Check sheet for the modelled part. Datum: model origin and axes. Units: mm. A direction names the side the tool comes from. Round coordinates to 2 decimals unless told otherwise and drop trailing zeros. Write each loop counter-clockwise with the first axis right and the second up, starting at its lowest first coordinate (ties: lowest second). Pieces come first, ordered by that corner, then holes. Notation, with made-up numbers: (-34, -23.75) -> (9, -23.75) arc R25 ccw to (9, 3.25) -> close; hole circle Ø10 at (36, 20.5). An arc over 180 degrees is marked (long way). One line per item, written item: value.
from build123d import *

# Parameters (mm, degrees)
SKETCH1_R           = 27.5
SKETCH1_R_2         = 17.5
BOSS_EXTRUDE1_DEPTH = 5
SKETCH2_W           = 120
SKETCH2_H           = 6
BOSS_EXTRUDE2_DEPTH = 10
SKETCH3_W           = 5
SKETCH3_H           = 3
CUT_EXTRUDE1_DEPTH  = 140
CHAMFER1_SIZE       = 5


with BuildPart() as part:
    # Sketch1 → Boss-Extrude1 (new body)
    with BuildSketch(Plane.XY):
        Circle(SKETCH1_R)
        Circle(SKETCH1_R_2, mode=Mode.SUBTRACT)
    extrude(amount=BOSS_EXTRUDE1_DEPTH)

    # Sketch2 → Boss-Extrude2 (add)
    with BuildSketch(Plane.XY.offset(5)):
        with Locations((77.5, 0)):
            Rectangle(SKETCH2_W, SKETCH2_H)
    extrude(amount=-BOSS_EXTRUDE2_DEPTH)

    # Sketch3 → Cut-Extrude1 (cut)
    with BuildSketch(Plane.ZY.offset(-17.5)):
        with Locations((-2.5, 1.5)):
            Rectangle(SKETCH3_W, SKETCH3_H)
    extrude(amount=-CUT_EXTRUDE1_DEPTH, mode=Mode.SUBTRACT)

    # Chamfer1
    chamfer1_edges = [part.edges().sort_by_distance(p)[0] for p in [
        (17.5, -1.5, -5),
    ]]
    chamfer(chamfer1_edges, length=CHAMFER1_SIZE - 0.0001)  # a hair under: the kernel refuses the full size


solid = part.part
Item 1: Sectioned sample at B-B on y = -12. Enter the section's corners in (x, z).
Answer:
outline: (-24.74, 0) -> (-12.74, 0) -> (-12.74, 5) -> (-24.74, 5) -> close; (12.74, 0) -> (24.74, 0) -> (24.74, 5) -> (12.74, 5) -> close
Item 2: Mould release check, pull along X, two halves, no side actions. Record for faces 4 (the flat face through (137.5, -1, 1)), 5 (the cylindrical face through (-13.887, -10.648, 2.465)), 6 (the cylindrical face through (-27.475, 1.167, 2.465)), 7 (the flat face through (79, -1, -5)): pulls with the +X half, pulls with the -X half, needs draft (parallel to the pull), parting line crosses it, or undercut.
Answer:
face 4: pulls with the +X half
face 5: undercut
face 6: parting line crosses it
face 7: needs draft
Item 3: Sectioned sample at A-A on x = 0. Enter the section's corners in (y, z), and give its area (3 significant figures).
Answer:
outline: (-27.5, 0) -> (-17.5, 0) -> (-17.5, 5) -> (-27.5, 5) -> close; (17.5, 0) -> (27.5, 0) -> (27.5, 5) -> (17.5, 5) -> close
area: 100 mm^2
Item 4: Sectioned sample at D-D on x = 122.5. Enter the section's corners in (y, z).
Answer:
outline: (-3, -5) -> (0, -5) -> (0, 0) -> (3, 0) -> (3, 5) -> (-3, 5) -> close
Item 5: Tool access check on faces 1 (the flat face through (82, 3, 3)), 2 (the flat face through (24, 0, 5)), 3 (the flat face through (77, 0, -3)). Record the directions out of +Z, -Z, +X, -X, +Y, -Y that give a thin tool (end or side, any length) a straight path to the whole face; none if there is none.
Answer:
face 1: +Z, -Z, +X, +Y
face 2: +Z, +X, -X, +Y, -Y
face 3: -Z, +X, -X, +Y
Item 6: Depth check by flat-ended pin: P1, Ø3, axis at x = 102, z = 3, coming from the -Y side; P2, Ø4, axis at x = 86.5, z = 1.5, coming from the +Y side; P3, Ø2, axis at y = -22, z = 3.5, coming from the +X side; P4, Ø1.5, axis at y = 6, z = -1.5, coming from the +X side. Enter the tip coordinate at first touch or a pass-through.
Answer:
P1: stops at y = -3
P2: stops at y = 3
P3: stops at x = 17.76
P4: passes through
Item 7: Thickness scan on line 1 (Y direction, x = 0, z = 2.25); line 2 (Y direction, x = 93, z = 4); line 3 (Y direction, x = -12, z = 0.75). Record the ranges inside material, lowest first.
Answer:
line 1: y = -27.5 to -17.5, 17.5 to 27.5
line 2: y = -3 to 3
line 3: y = -24.74 to -12.74, 12.74 to 24.74
Item 8: Sectioned sample at C-C on z = 1.75. Enter the section's corners in (x, y), and give its area (3 significant figures).
Answer:
outline: (27.34, -3) -> (137.5, -3) -> (137.5, 3) -> (27.34, 3) arc R27.5 ccw (long way) to start; hole circle Ø35 at (0, 0)
area: 2,070 mm^2
